Part model, mm, in its own coordinate system. A direction names the side the tool comes from. Give positions to 0.01 mm unless a question says otherwise; leave off trailing zeros. Write each loop counter-clockwise with the first axis right and the second up, starting at its lowest first coordinate (ties: lowest second). Pieces come first, ordered by that corner, then holes. Notation, with made-up numbers: M 69,-27.75 L 106,-27.75 A22 ccw 106,-5.75 Z; hole C 34.25,-24.5 d3. An arc over 180 degrees is marked long. Use a Markdown table: item, result. Add a question column.
from build123d import *

# Parameters (mm, degrees)
BOSS_EXTRUDE1_DEPTH = 130
SKETCH3_W           = 75.312470342
SKETCH3_H           = 30
CUT_EXTRUDE1_DEPTH  = 14
SKETCH4_W           = 75.312470342
SKETCH4_H           = 60
CUT_EXTRUDE2_DEPTH  = 14
SKETCH5_W           = 6
SKETCH5_H           = 8
CUT_EXTRUDE3_DEPTH  = 94
SKETCH6_W           = 6
SKETCH6_H           = 8
CUT_EXTRUDE4_DEPTH  = 94


with BuildPart() as part:
    # Sketch1 → Boss-Extrude1 (new body)
    with BuildSketch(Plane.XY):
        Polygon((37.656235171, 16), (-37.656235171, 16), (-37.656235171, 2), (-17.656235171, 2), (-17.656235171, -8), (-26.236747462, -8), (-26.236747462, -16), (26.236747462, -16), (26.236747462, -8), (17.656235171, -8), (17.656235171, 2), (37.656235171, 2), align=None)
    extrude(amount=BOSS_EXTRUDE1_DEPTH)

    # Sketch3 → Cut-Extrude1 (cut)
    with BuildSketch(Plane(origin=(0, 16, 0), x_dir=(1, 0, 0), z_dir=(0, 1, 0))):
        with Locations((0, -95)):
            Rectangle(SKETCH3_W, SKETCH3_H)
    extrude(amount=-CUT_EXTRUDE1_DEPTH, mode=Mode.SUBTRACT)

    # Sketch4 → Cut-Extrude2 (cut)
    with BuildSketch(Plane(origin=(0, 16, 0), x_dir=(1, 0, 0), z_dir=(0, 1, 0))):
        with Locations((0, -30)):
            Rectangle(SKETCH4_W, SKETCH4_H)
    extrude(amount=-CUT_EXTRUDE2_DEPTH, mode=Mode.SUBTRACT)

    # Sketch5 → Cut-Extrude3 (cut)
    with BuildSketch(Plane.ZY.offset(37.656235171)):
        with Locations((77, 6)):
            Rectangle(SKETCH5_W, SKETCH5_H)
    extrude(amount=-CUT_EXTRUDE3_DEPTH, mode=Mode.SUBTRACT)

    # Sketch6 → Cut-Extrude4 (cut)
    with BuildSketch(Plane.ZY.offset(37.656235171)):
        with Locations((113, 6)):
            Rectangle(SKETCH6_W, SKETCH6_H)
    extrude(amount=-CUT_EXTRUDE4_DEPTH, mode=Mode.SUBTRACT)


solid = part.part
1. Cut at C-C (y = 5). Write the cut outline in (x, z).
2. Cut at A-A (y = 13). Write the cut outline in (x, z).
3. Cut at D-D (x = 12). Write the cut outline in (y, z).
4. Cut at B-B (x = 28). Write the cut outline in (y, z).
5. Mould opens along Z. For faces 6 (the flat face through (-1, 0, 130)), 7 (the flat face through (0, -7, 0)), 8 (the flat face through (-1, 10, 113)), 9 (the flat face through (-28, 2, 123)) say: released by +Z, released by -Z, zero draft, split by the parting line, or undercut.
6. Tool access for faces 1 (the flat face through (28, 2, 67)), 2 (the flat face through (26.237, -12, 64)), 3 (the flat face through (-1, 6, 116)), 4 (the flat face through (0, 2, 30)), 5 (the flat face through (-1, 13, 80)): list every direction of +Z, -Z, +X, -X, +Y, -Y with a clear straight run to the whole face (end or side of a thin tool).
7. Drill centre lines: probe 1 along Z at (x, y) = (1.5, 12); probe 2 along Z at (x, y) = (-10, 5.5); probe 3 along Y at (x, z) = (-14, 98.5). Where is each one in solid material? Low to high. Write a range as [from, to].
8. Flat gauge pins, fed straight in: pin 1 (2.5 mm diameter, centred on x = -20, z = 43, fed in from +Y); pin 2 (8 mm diameter, centred on x = 21, z = 92, fed in from +Y); pin 3 (2.5 mm diameter, centred on x = -2, y = 6, fed in from -Z). Where does each tip first touch, or does it go through?
A:
| question | item | result |
|---|---|---|
| 1 | outline | M -37.66,60 L 37.66,60 L 37.66,74 L -37.66,74 Z; M -37.66,116 L 37.66,116 L 37.66,130 L -37.66,130 Z |
| 2 | outline | M -37.66,60 L 37.66,60 L 37.66,80 L -37.66,80 Z; M -37.66,110 L 37.66,110 L 37.66,130 L -37.66,130 Z |
| 3 | outline | M -16,0 L 2,0 L 2,60 L 16,60 L 16,80 L 10,80 L 10,74 L 2,74 L 2,116 L 10,116 L 10,110 L 16,110 L 16,130 L -16,130 Z |
| 4 | outline | M 2,60 L 16,60 L 16,80 L 10,80 L 10,74 L 2,74 Z; M 2,116 L 10,116 L 10,110 L 16,110 L 16,130 L 2,130 Z |
| 5 | face 6 | released by +Z |
| 5 | face 7 | released by -Z |
| 5 | face 8 | undercut |
| 5 | face 9 | zero draft |
| 6 | face 1 | +Z, -Z, +X |
| 6 | face 2 | +Z, -Z, +X, -Y |
| 6 | face 3 | +X, -X |
| 6 | face 4 | -Z, +X, -X, +Y |
| 6 | face 5 | +X, -X, +Y |
| 7 | probe 1 | z = [60, 80], [110, 130] |
| 7 | probe 2 | z = [60, 74], [116, 130] |
| 7 | probe 3 | y = [-16, 2] |
| 8 | pin 1 | stops at y = -8 |
| 8 | pin 2 | stops at y = 2 |
| 8 | pin 3 | stops at z = 60 |
